```python
from build123d import *


with BuildPart() as f2:
    # F2: sweep along a path in F0
    with BuildLine(Plane.XZ) as f2_path:
        Line((0, 0), (2000, 0))
        Line((2000, 0), (2000, 700))
        Line((2000, 700), (0, 700))
        Line((0, 700), (0, 0))
    # F1 (on Right) → F2 (sweep)
    with BuildSketch(Plane.YZ):
        Polygon((-45, 0), (0, 0), (45, 0), (45, 40), (33, 40), (33, 37), (42, 37), (42, 3), (0, 3), (-42, 3), (-42, 37), (-33, 37), (-33, 40), (-45, 40), align=None)
    sweep(path=f2_path.line, transition=Transition.RIGHT)


solid = f2.part
```
Input: part model. Units: mm. Frame: model coordinates. A direction names the side the tool comes from. Give positions to 0.01 mm unless a question says otherwise; leave off trailing zeros. Order: outer loops, then holes, each group sorted by start corner. A loop starts at its lowest first (then second) coordinate and runs counter-clockwise, first axis right, second up.
1. Section B-B on x = 1058.5. Return the cut outline in (y, z), and give its area (3 significant figures).
Derived:
outline: (-45, 0) - (45, 0) - (45, 40) - (33, 40) - (33, 37) - (42, 37) - (42, 3) - (-42, 3) - (-42, 37) - (-33, 37) - (-33, 40) - (-45, 40) - close; (-45, 660) - (-33, 660) - (-33, 663) - (-42, 663) - (-42, 697) - (42, 697) - (42, 663) - (33, 663) - (33, 660) - (45, 660) - (45, 700) - (-45, 700) - close
area: 1,090 mm2
2. Material intervals for L1, parallel to Z at x = 550, y = 37; L2, parallel to X at y = -16, z = 183.5; L3, parallel to Z at x = 1665, y = -18, sorted ascending.
Derived:
L1: z = 0 to 3, 37 to 40, 660 to 663, 697 to 700
L2: x = 0 to 3, 1997 to 2000
L3: z = 0 to 3, 697 to 700
3. Section C-C on z = 82.5. Return the cut outline in (x, y).
Derived:
outline: (0, -45) - (40, -45) - (40, -33) - (37, -33) - (37, -42) - (3, -42) - (3, 42) - (37, 42) - (37, 33) - (40, 33) - (40, 45) - (0, 45) - close; (1960, -45) - (2000, -45) - (2000, 45) - (1960, 45) - (1960, 33) - (1963, 33) - (1963, 42) - (1997, 42) - (1997, -42) - (1963, -42) - (1963, -33) - (1960, -33) - close
4. Section A-A on y = -9. Return the cut outline in (x, z).
Derived:
outline: (0, 0) - (2000, 0) - (2000, 700) - (0, 700) - close; hole (3, 3) - (1997, 3) - (1997, 697) - (3, 697) - close
5. Mould query, pull axis Z, two halves, no side actions, for faces 3 (the flat face through (1014, -1, 0)), 4 (the flat face through (1997, 1, 355)), 5 (the flat face through (1227, -45, 663)). Classes: released by +Z, released by -Z, zero draft, split by the parting line, or undercut.
Derived:
face 3: released by -Z
face 4: undercut
face 5: zero draft
6. Reachability of faces 1 (the flat face through (0, -1, 345)), 2 (the flat face through (1300, 42, 686)) from +Z, -Z, +X, -X, +Y, -Y: full face, straight path, thin tool, end or side. Return the list, or none.
Derived:
face 1: +Z, -Z, -X, +Y, -Y
face 2: none
